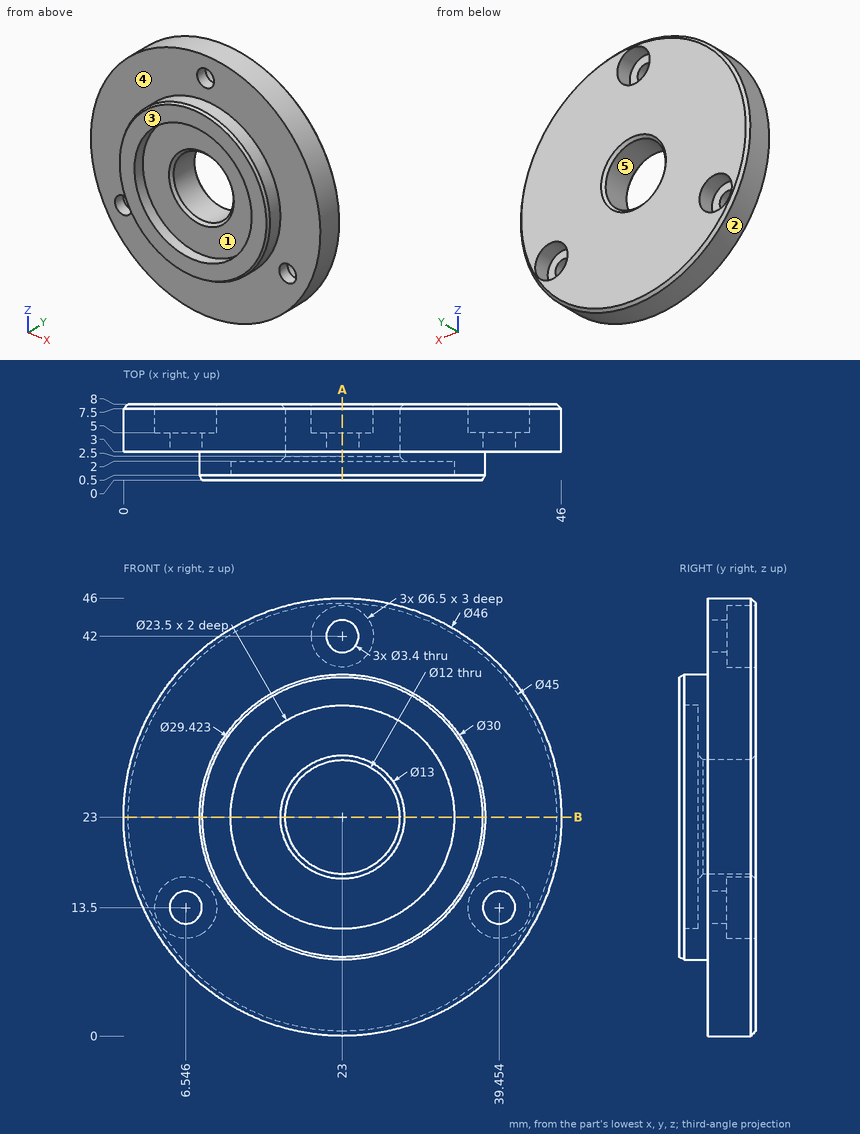
Answer from the drawing. Dimensions are ordinates in mm from the lowest x, y and z of the part. A direction names the side the tool comes from. Round coordinates to 2 decimals unless told otherwise and drop trailing zeros. Order: outer loops, then holes, each group sorted by start corner. A loop starts at its lowest first (then second) coordinate and runs counter-clockwise, first axis right, second up.
1) The mould has two halves that part along Z. Classify the marked faces 1, 2 and 3: released by +Z, released by -Z, zero draft, split by the parting line, or undercut.
2) Flat-ended cylindrical pins translate along their axes: pin 1 (6 mm diameter, centred on x = 23, z = 42, fed in from -Y); pin 2 (12 mm diameter, centred on x = 24, z = 26, fed in from -Y); pin 3 (3 mm diameter, centred on y = 6.5, z = 35, fed in from -X); pin 4 (2.5 mm diameter, centred on x = 39.45, z = 13.5, fed in from +Y). Find the tip coordinate at first contact, or state that the pin passes through.
3) The part is cut by section A-A on x = 23. Give the number of separate pieces and of enclosed holes in the cut face, plus the area to 3 significant figures.
4) The part is cut by section B-B on z = 23. Write down the section's boundary in (x, y).
5) Straight lines are drawn through the part: L1, parallel to X at y = 6.35, z = 23; L2, parallel to X at y = 7, z = 10.5 (1 decimal); L3, parallel to Y at x = 23, z = 39. For each, find the intervals that lie inside material, in ascending order.
6) For the marked faces 4 and 5, determine the directions among +Z, -Z, +X, -X, +Y, -Y from which every point of the face is accessible in a straight line to the end or side of a thin tool.
Resolved:
1. face 1: undercut
1. face 2: split by the parting line
1. face 3: zero draft
2. pin 1: stops at y = 3
2. pin 2: stops at y = 2
2. pin 3: stops at x = 2.54
2. pin 4: passes through
3. separate pieces: 3
3. enclosed holes: 0
3. area: 174 mm2
4. outline: (0, 3) - (8, 3) - (8, 0.5) - (8.29, 0) - (11.25, 0) - (11.25, 2) - (16.5, 2) - (17, 2.5) - (17, 7.5) - (16.5, 8) - (0.5, 8) - (0, 7.5) - close; (29, 2.5) - (29.5, 2) - (34.75, 2) - (34.75, 0) - (37.71, 0) - (38, 0.5) - (38, 3) - (46, 3) - (46, 7.5) - (45.5, 8) - (29.5, 8) - (29, 7.5) - close
5. L1: x = 0 to 17, 29 to 46
5. L2: x = 3.7 to 5.3, 7.8 to 38.2, 40.7 to 42.3
5. L3: y = 3 to 5
6. face 4: -Y
6. face 5: +Y, -Y
